from build123d import *

# Parameters (mm, degrees)
SKETCH1_R           = 1.5
SKETCH1_R_2         = 1.75
BOSS_EXTRUDE3_DEPTH = 2
CUT_EXTRUDE1_DEPTH  = 2
FILLET1_R           = 1
SCALE1_SCALE        = 2


with BuildPart() as part:
    # Sketch1 → Boss-Extrude3 (new body)
    with BuildSketch(Plane(origin=(0, 0, 0), x_dir=(1, 0, 0), z_dir=(0, 1, 0))):
        with BuildLine():
            Line((6.048353149, 16.421553647), (2.27592576, 17.351373488))
            ThreePointArc((2.27592576, 17.351373488), (1.69730064, 18.342788524), (1.499767326, 19.473580897))
            ThreePointArc((1.499767326, 19.473580897), (1.49994183, 19.486789936), (1.5, 19.5))
            ThreePointArc((1.5, 19.5), (0, 21), (-1.5, 19.5))
            ThreePointArc((-1.5, 19.5), (-1.49994183, 19.486789936), (-1.499767326, 19.473580897))
            ThreePointArc((-1.499767326, 19.473580897), (-1.69730064, 18.342788524), (-2.27592576, 17.351373488))
            Line((-2.27592576, 17.351373488), (-6.048353149, 16.421553647))
            ThreePointArc((-6.048353149, 16.421553647), (-7.021433788, 17.030507563), (-7.72184627, 17.939976175))
            ThreePointArc((-7.72184627, 17.939976175), (-7.7278303, 17.951753295), (-7.733917816, 17.963477258))
            ThreePointArc((-7.733917816, 17.963477258), (-9.759186613, 18.594576539), (-10.390285893, 16.569307742))
            ThreePointArc((-10.390285893, 16.569307742), (-10.384020417, 16.557678026), (-10.377802301, 16.546022918))
            ThreePointArc((-10.377802301, 16.546022918), (-10.027203946, 15.452957688), (-10.078817505, 14.30620277))
            Line((-10.078817505, 14.30620277), (-12.987027242, 11.729753767))
            ThreePointArc((-12.987027242, 11.729753767), (-14.131642352, 11.81674256), (-15.174477944, 12.296539112))
            ThreePointArc((-15.174477944, 12.296539112), (-15.18524964, 12.304186316), (-15.196088265, 12.31173836))
            ThreePointArc((-15.196088265, 12.31173836), (-17.282661184, 11.929359681), (-16.900282505, 9.842786762))
            ThreePointArc((-16.900282505, 9.842786762), (-16.889330102, 9.835400872), (-16.878407836, 9.827970489))
            ThreePointArc((-16.878407836, 9.827970489), (-16.059995669, 9.023040475), (-15.572773623, 7.983653406))
            Line((-15.572773623, 7.983653406), (-16.950529904, 4.350808657))
            ThreePointArc((-16.950529904, 4.350808657), (-18.004461959, 3.895904243), (-19.150819593, 3.836113127))
            ThreePointArc((-19.150819593, 3.836113127), (-19.163911289, 3.837878533), (-19.177018025, 3.839528576))
            ThreePointArc((-19.177018025, 3.839528576), (-20.846886356, 2.531270285), (-19.538628065, 0.861401954))
            ThreePointArc((-19.538628065, 0.861401954), (-19.5254978, 0.859951908), (-19.512373542, 0.858448461))
            ThreePointArc((-19.512373542, 0.858448461), (-18.413635928, 0.526053428), (-17.499194975, -0.167854741))
            Line((-17.499194975, -0.167854741), (-17.030870442, -4.024854283))
            ThreePointArc((-17.030870442, -4.024854283), (-17.752676308, -4.917438785), (-18.739939265, -5.503120145))
            ThreePointArc((-18.739939265, -5.503120145), (-18.752351812, -5.50764097), (-18.764724063, -5.512270933))
            ThreePointArc((-18.764724063, -5.512270933), (-19.635341096, -7.446702628), (-17.700909402, -8.317319661))
            ThreePointArc((-17.700909402, -8.317319661), (-17.688609259, -8.312501675), (-17.676289619, -8.307733764))
            ThreePointArc((-17.676289619, -8.307733764), (-16.548934104, -8.09144612), (-15.416761648, -8.280909389))
            Line((-15.416761648, -8.280909389), (-13.209643805, -11.478471612))
            ThreePointArc((-13.209643805, -11.478471612), (-13.433966457, -12.604255849), (-14.035964693, -13.581654911))
            ThreePointArc((-14.035964693, -13.581654911), (-14.044854525, -13.591426301), (-14.053657958, -13.601275602))
            ThreePointArc((-14.053657958, -13.601275602), (-13.925575823, -15.718725712), (-11.808125713, -15.590643577))
            ThreePointArc((-11.808125713, -15.590643577), (-11.799473508, -15.5806613), (-11.790780767, -15.570714303))
            ThreePointArc((-11.790780767, -15.570714303), (-10.893070914, -14.855292874), (-9.802534018, -14.496907492))
            Line((-9.802534018, -14.496907492), (-6.362246966, -16.302509425))
            ThreePointArc((-6.362246966, -16.302509425), (-6.037696789, -17.403589796), (-6.116519761, -18.548796214))
            ThreePointArc((-6.116519761, -18.548796214), (-6.119850325, -18.561579661), (-6.12306818, -18.574391943))
            ThreePointArc((-6.12306818, -18.574391943), (-5.02562895, -20.389778166), (-3.210242727, -19.292338936))
            ThreePointArc((-3.210242727, -19.292338936), (-3.207220575, -19.279479189), (-3.204146136, -19.266631842))
            ThreePointArc((-3.204146136, -19.266631842), (-2.741736452, -18.215971056), (-1.942663979, -17.391838795))
            Line((-1.942663979, -17.391838795), (1.942663979, -17.391838795))
            ThreePointArc((1.942663979, -17.391838795), (2.741736452, -18.215971056), (3.204146136, -19.266631842))
            ThreePointArc((3.204146136, -19.266631842), (3.207137832, -19.279498812), (3.210242727, -19.292338936))
            ThreePointArc((3.210242727, -19.292338936), (5.02562895, -20.389778166), (6.12306818, -18.574391943))
            ThreePointArc((6.12306818, -18.574391943), (6.11976794, -18.561600739), (6.116519761, -18.548796214))
            ThreePointArc((6.116519761, -18.548796214), (6.037696789, -17.403589796), (6.362246966, -16.302509425))
            Line((6.362246966, -16.302509425), (9.802534018, -14.496907492))
            ThreePointArc((9.802534018, -14.496907492), (10.893070914, -14.855292874), (11.790780767, -15.570714303))
            ThreePointArc((11.790780767, -15.570714303), (11.799409362, -15.580717128), (11.808125713, -15.590643577))
            ThreePointArc((11.808125713, -15.590643577), (13.925575823, -15.718725712), (14.053657958, -13.601275602))
            ThreePointArc((14.053657958, -13.601275602), (14.044791371, -13.591483251), (14.035964693, -13.581654911))
            ThreePointArc((14.035964693, -13.581654911), (13.433966458, -12.604255849), (13.209643805, -11.478471612))
            Line((13.209643805, -11.478471612), (15.416761648, -8.280909389))
            ThreePointArc((15.416761648, -8.280909389), (16.548934104, -8.09144612), (17.676289619, -8.307733764))
            ThreePointArc((17.676289619, -8.307733764), (17.688578405, -8.312580919), (17.700909402, -8.317319661))
            ThreePointArc((17.700909402, -8.317319661), (19.635341096, -7.446702628), (18.764724063, -5.512270933))
            ThreePointArc((18.764724063, -5.512270933), (18.752322358, -5.507720745), (18.739939265, -5.503120145))
            ThreePointArc((18.739939265, -5.503120145), (17.752676308, -4.917438785), (17.030870442, -4.024854283))
            Line((17.030870442, -4.024854283), (17.499194975, -0.167854741))
            ThreePointArc((17.499194975, -0.167854741), (18.413635928, 0.526053428), (19.512373542, 0.858448461))
            ThreePointArc((19.512373542, 0.858448461), (19.525507306, 0.859867402), (19.538628065, 0.861401954))
            ThreePointArc((19.538628065, 0.861401954), (20.846886356, 2.531270285), (19.177018025, 3.839528576))
            ThreePointArc((19.177018025, 3.839528576), (19.163922282, 3.837794208), (19.150819593, 3.836113127))
            ThreePointArc((19.150819593, 3.836113127), (18.004461959, 3.895904243), (16.950529904, 4.350808657))
            Line((16.950529904, 4.350808657), (15.572773623, 7.983653406))
            ThreePointArc((15.572773623, 7.983653406), (16.059995669, 9.023040475), (16.878407836, 9.827970489))
            ThreePointArc((16.878407836, 9.827970489), (16.889377792, 9.835330464), (16.900282505, 9.842786762))
            ThreePointArc((16.900282505, 9.842786762), (17.282661184, 11.929359681), (15.196088265, 12.31173836))
            ThreePointArc((15.196088265, 12.31173836), (15.185298562, 12.304116759), (15.174477944, 12.296539112))
            ThreePointArc((15.174477944, 12.296539112), (14.131642352, 11.81674256), (12.987027242, 11.729753767))
            Line((12.987027242, 11.729753767), (10.078817505, 14.30620277))
            ThreePointArc((10.078817505, 14.30620277), (10.027203946, 15.452957688), (10.377802301, 16.546022918))
            ThreePointArc((10.377802301, 16.546022918), (10.384095364, 16.557637845), (10.390285893, 16.569307742))
            ThreePointArc((10.390285893, 16.569307742), (9.759186613, 18.594576539), (7.733917816, 17.963477258))
            ThreePointArc((7.733917816, 17.963477258), (7.727905944, 17.95171444), (7.72184627, 17.939976175))
            ThreePointArc((7.72184627, 17.939976175), (7.021433788, 17.030507563), (6.048353149, 16.421553647))
        make_face()
        with Locations(Location((0, -9, 0), (0, 0, 270))):
            Circle(SKETCH1_R, mode=Mode.SUBTRACT)
        with Locations(Location((-7.794228634, -4.5, 0), (0, 0, 270))):
            Circle(SKETCH1_R, mode=Mode.SUBTRACT)
        with Locations(Location((0, 0, 0), (0, 0, 270))):
            Circle(SKETCH1_R_2, mode=Mode.SUBTRACT)
        with Locations(Location((7.794228634, -4.5, 0), (0, 0, 270))):
            Circle(SKETCH1_R, mode=Mode.SUBTRACT)
        with Locations(Location((-7.794228634, 4.5, 0), (0, 0, 270))):
            Circle(SKETCH1_R, mode=Mode.SUBTRACT)
        with Locations(Location((0, 9, 0), (0, 0, 270))):
            Circle(SKETCH1_R, mode=Mode.SUBTRACT)
        with Locations(Location((7.794228634, 4.5, 0), (0, 0, 270))):
            Circle(SKETCH1_R, mode=Mode.SUBTRACT)
    extrude(amount=BOSS_EXTRUDE3_DEPTH)

    # Sketch3 → Cut-Extrude1 (cut)
    with BuildSketch(Plane(origin=(0, 2, 0), x_dir=(1, 0, 0), z_dir=(0, 1, 0))):
        with BuildLine():
            Line((-3, 14.186260959), (-3, 11.618950039))
            ThreePointArc((-3, 11.618950039), (-10.392304845, 6), (-11.562305899, -3.211398808))
            Line((-11.562305899, -3.211398808), (-13.785662375, -4.495054268))
            ThreePointArc((-13.785662375, -4.495054268), (-12.557368355, 7.25), (-3, 14.186260959))
        make_face()
        with BuildLine():
            Line((3, 14.186260959), (3, 11.618950039))
            ThreePointArc((3, 11.618950039), (10.392304845, 6), (11.562305899, -3.211398808))
            Line((11.562305899, -3.211398808), (13.785662375, -4.495054268))
            ThreePointArc((13.785662375, -4.495054268), (12.557368355, 7.25), (3, 14.186260959))
        make_face()
        with BuildLine():
            Line((10.785662375, -9.691206691), (8.562305899, -8.407551231))
            ThreePointArc((8.562305899, -8.407551231), (0, -12), (-8.562305899, -8.407551231))
            Line((-8.562305899, -8.407551231), (-10.785662375, -9.691206691))
            ThreePointArc((-10.785662375, -9.691206691), (0, -14.5), (10.785662375, -9.691206691))
        make_face()
    extrude(amount=-CUT_EXTRUDE1_DEPTH, mode=Mode.SUBTRACT)

    # Fillet1
    fillet1_edges = [part.edges().sort_by_distance(p)[0] for p in [
        (-8.562305899, 1, 8.407551231),
        (8.562305899, 1, 8.407551231),
        (10.785662375, 1, 9.691206691),
        (-10.785662375, 1, 9.691206691),
        (11.562305899, 1, 3.211398808),
        (3, 1, -11.618950039),
        (3, 1, -14.186260959),
        (13.785662375, 1, 4.495054268),
        (-3, 1, -11.618950039),
        (-11.562305899, 1, 3.211398808),
        (-13.785662375, 1, 4.495054268),
        (-3, 1, -14.186260959),
    ]]
    fillet(fillet1_edges, radius=FILLET1_R)


with BuildPart() as part_1:
    # Scale1: scaled about (0, 0, 0)
    add(part.part.scale(SCALE1_SCALE))


solid = part_1.part
The listing builds one solid part. Answer for the finished solid, in the listing's coordinates (mm). A direction names the side the tool comes from. Coordinates: 2 decimals unless noted, no trailing zeros. Loops run counter-clockwise (first coordinate to the right, second up) from the corner with the lowest first, then second, coordinate; pieces in that order, holes last. Notation, with made-up numbers: (21, -12) -> (31, -12) arc R17 cw to (31, 14) -> close; hole circle Ø3 at (59, 45.25). An arc over 180 degrees is marked (long way). Answer in a Markdown table with one row per item. Add a question column.
1. The part is cut by section A-A, the plane x = 0. Write down the section's boundary in (y, z).
2. The part is cut by section C-C, the plane y = 0.6. Count the separate pieces of the cut face and the enclosed holes in it, then the cut area to 3 significant figures.
3. Determine the mould class of faces 1 (the cylindrical face through (5.47, 1.97, 36.41)), 2 (the cylindrical face through (-27.158, 1.972, 7.787)), 3 (the cylindrical face through (-28.232, 1.972, -23.625)) for opening direction Z: +Z half, -Z half, draft (parallel to the pull), parting line (faces both ways), or undercut.
4. Consider line 1 (X direction, y = 1.9, z = 0); line 2 (X direction, y = 2, z = 9); line 3 (Z direction, x = -7, y = 1.65). Determine where each line is inside the solid, lowest interval first. Write a range as [from, to].
5. The part is cut by section B-B, the plane z = -18. Write down the section's boundary in (x, y).
6. For faces 4 (the flat face through (8.38, 1.97, -33.76)), 5 (the cylindrical face through (-21.815, 1.972, 29.726)), 6 (the cylindrical face through (12.07, 1.97, 34.84)), 7 (the cylindrical face through (0, 2, 24)), determine the directions among +Z, -Z, +X, -X, +Y, -Y from which every point of the face is accessible in a straight line to the end or side of a thin tool.
7. Flat-ended cylindrical pins translate along their axes: P1, Ø6.5, axis at x = 0, z = 0, coming from the +Y side; P2, Ø2, axis at x = 0.5, y = 2, coming from the +Z side; P3, Ø0.5, axis at y = 2, z = -25.5, coming from the -X side; P4, Ø2, axis at x = -31.5, y = 1, coming from the -Z side. Find the tip coordinate at first contact, or state that the pin passes through.
Answer below:
| question | item | result |
|---|---|---|
| 1 | outline | (0, -42) -> (4, -42) -> (4, -21) -> (0, -21) -> close; (0, -15) -> (4, -15) -> (4, -3.5) -> (0, -3.5) -> close; (0, 3.5) -> (4, 3.5) -> (4, 15) -> (0, 15) -> close; (0, 21) -> (4, 21) -> (4, 24) -> (0, 24) -> close; (0, 29) -> (4, 29) -> (4, 34.78) -> (0, 34.78) -> close |
| 2 | separate pieces | 1 |
| 2 | enclosed holes | 10 |
| 2 | area | 3,540 mm2 |
| 3 | face 1 | +Z half |
| 3 | face 2 | undercut |
| 3 | face 3 | -Z half |
| 4 | line 1 | [-35.33, -29], [-24, -3.5], [3.5, 24], [29, 35.33] |
| 4 | line 2 | [-34.7, -18.59], [-12.59, 12.59], [18.59, 34.7] |
| 4 | line 3 | [-34.1, -27.52], [-23.01, 22.96], [28.14, 39.75] |
| 5 | outline | (-32.09, 0) -> (-22.74, 0) -> (-22.74, 4) -> (-32.09, 4) -> close; (-15.87, 0) -> (-3, 0) -> (-3, 4) -> (-15.87, 4) -> close; (3, 0) -> (15.87, 0) -> (15.87, 4) -> (3, 4) -> close; (22.74, 0) -> (32.09, 0) -> (32.09, 4) -> (22.74, 4) -> close |
| 6 | face 4 | -Z, +Y, -Y |
| 6 | face 5 | +Z, +Y, -Y |
| 6 | face 6 | +X, +Y, -Y |
| 6 | face 7 | +Y, -Y |
| 7 | P1 | through |
| 7 | P2 | z = 34.78 |
| 7 | P3 | x = -23.95 |
| 7 | P4 | z = -25.15 |
